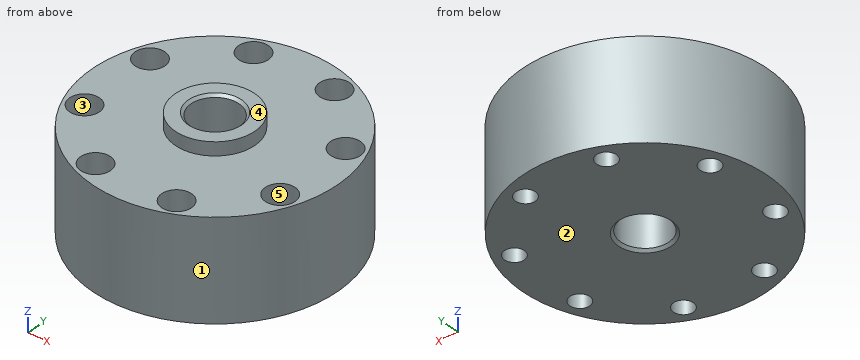
from build123d import *

# Parameters (mm, degrees)
ESBO_O1_R                = 37
RESSALTO_EXTRUS_O1_DEPTH = 30
FURO1_D                  = 6
FURO1_CBORE_D            = 9
FURO1_CBORE_DEPTH        = 7
PADR_OCIRCULAR1_COUNT    = 8
ESBO_O4_R                = 12
RESSALTO_EXTRUS_O2_DEPTH = 4


with BuildPart() as part:
    # Esbo_o1 → Ressalto-extrus_o1 (new body)
    with BuildSketch(Plane.XY):
        Circle(ESBO_O1_R)
    extrude(amount=RESSALTO_EXTRUS_O1_DEPTH)

    # Furo1 (through all)
    with Locations(Plane(origin=(-12.05452812, 29.102205274, 30), x_dir=(1, 0, 0), z_dir=(0, 0, 1))):
        with Locations((0, 0)):
            furo1 = CounterBoreHole(FURO1_D / 2, FURO1_CBORE_D / 2, FURO1_CBORE_DEPTH)

    # Padr_oCircular1: Furo1 ×8 about axis
    padr_ocircular1_axis = Axis((0, 0, 0), (0, 0, 1))
    for i in range(1, PADR_OCIRCULAR1_COUNT):
        add(furo1.rotate(padr_ocircular1_axis, i * 360 / PADR_OCIRCULAR1_COUNT), mode=Mode.SUBTRACT)

    # Esbo_o4 → Ressalto-extrus_o2 (add)
    with BuildSketch(Plane.XY.offset(30)):
        Circle(ESBO_O4_R)
    extrude(amount=RESSALTO_EXTRUS_O2_DEPTH)

    # Esbo_o7 → Furo roscado de M16x1.51 (revolve, cut)
    with BuildSketch(Plane(origin=(0, 0, 34), x_dir=(0, -1, 0), z_dir=(1, 0, 0))):
        Polygon((0, 0), (0, 34), (8.025, 34), (7.25, 33.225), (7.25, 0.775), (8.025, 0), align=None)
    revolve(axis=Axis((0, 0, 40.35), (0, 0, -1)), mode=Mode.SUBTRACT)


solid = part.part
Here's how the part is built. I have some questions about the finished solid (model axes, mm). Face numbers are marked on the shaded views. A direction names the side the tool comes from. Give positions to 0.01 mm unless a question says otherwise; leave off trailing zeros. Write each loop counter-clockwise with the first axis right and the second up, starting at its lowest first coordinate (ties: lowest second). Pieces come first, ordered by that corner, then holes. Notation, with made-up numbers: (30.25, 89.5) -> (57.25, 89.5) arc R33 ccw to (57.25, 121.5) -> close; hole circle Ø10 at (84, -12). An arc over 180 degrees is marked (long way). Use one line per item in the form item = value. Start each with the question number.
1. Imagine slicing it at D-D on x = 20. List the corners of the cut face in (y, z) for me.
2. Will these pins go through, and if not, where does the flat tip stop? pin 1 Ø2 at (y, z) = (20.5, 11) entering from +X; pin 2 Ø7 at (x, y) = (10.5, 27) entering from +Z; pin 3 Ø10 at (y, z) = (-12, 10) entering from +X.
3. Imagine slicing it at B-B on z = 26. State how many separate pieces and enclosed holes the cut face has, plus the area to 3 significant figures.
4. Imagine slicing it at A-A on x = 0. List the corners of the cut face in (y, z) for me (3 decimals).
5. If I drill on L1, parallel to X at y = 27.5, z = 17; L2, parallel to Y at x = 0, z = 17; L3, parallel to X at y = -28.5, z = 17.5, over which ranges is the centre line in solid material (lowest first)?
6. On a 3-axis mill with a long thin cutter (end or side, diameter ignored), from which of +Z, -Z, +X, -X, +Y, -Y can I reach the whole of each face in a straight line? I mean the marked faces 4 and 5. Say none if no direction works.
7. Thinking about a two-plate mould opening in X: for the marked faces 1, 2 and 3, which applies, +X half, -X half, draft (parallel to the pull), parting line (faces both ways), or undercut?
Entries:
q1.outline = (-31.13, 0) -> (31.13, 0) -> (31.13, 30) -> (-31.13, 30) -> close
q2.pin_1 = 31.44
q2.pin_2 = 30
q2.pin_3 = 36.33
q3.separate_pieces = 1
q3.enclosed_holes = 9
q3.area = 3,630 mm²
q4.outline = (-37, 0) -> (-8.025, 0) -> (-7.25, 0.775) -> (-7.25, 33.225) -> (-8.025, 34) -> (-12, 34) -> (-12, 30) -> (-37, 30) -> close; (7.25, 0.775) -> (8.025, 0) -> (37, 0) -> (37, 30) -> (12, 30) -> (12, 34) -> (8.025, 34) -> (7.25, 33.225) -> close
q5.L1 = -24.75 to -14.59, -9.52 to 9.52, 14.59 to 24.75
q5.L2 = -37 to -7.25, 7.25 to 37
q5.L3 = -23.6 to -14.99, -9.12 to 9.12, 14.99 to 23.6
q6.face_4 = +Z, +X, -X, +Y, -Y
q6.face_5 = +Z
q7.face_1 = parting line
q7.face_2 = draft
q7.face_3 = undercut
